Autodesk Fusion 360 part; units mm, degrees
sketch "Boceto1" plane through (0, 0, 0) normal (0, 0, 1) x (1, 0, 0)
  circle A0 centre (0, 0) radius 11.5
  line L0 (0, 0) -> (11.5, 0)
  line L1 (0, 0) -> (5.75, 9.9593)
  line L2 (0, 0) -> (-5.75, 9.9593)
  line L3 (0, 0) -> (-11.5, 0)
  line L4 (0, 0) -> (-5.75, -9.9593)
  line L5 (0, 0) -> (5.75, -9.9593)
  line L6 (5.75, 9.9593) -> (-5.75, 9.9593)
  line L7 (-5.75, 9.9593) -> (-11.5, 0)
  line L8 (-11.5, 0) -> (-5.75, -9.9593)
  line L9 (-5.75, -9.9593) -> (5.75, -9.9593)
  line L10 (5.75, -9.9593) -> (11.5, 0)
  line L11 (11.5, 0) -> (5.75, 9.9593)
  circle A1 centre (0, 0) radius 14
  dimension "d1" = 23
  dimension "d3" = 360
  dimension "d5" = 360
  dimension "d6" = 28
extrude "Extruir1" add sketch "Boceto1" along normal blind 24 contours A0 L11 | A0 L10 | A0 L6 | A0 L9 | A0 L7 | A0 L8 | A1
sketch "Boceto2" plane through (8.625, 4.9796, 0) normal (-0.866, -0.5, 0) x (0.5, -0.866, 0)
  line L0 (-5.75, 0) -> (5.75, 0)
  line L1 (5.75, 0) -> (5.75, 24)
  line L2 (5.75, 24) -> (-5.75, 24)
  line L3 (-5.75, 24) -> (-5.75, 0)
  circle A0 centre (0.25, 17) radius 4.5
  dimension "d9" = 9
  dimension "d10" = 7
  dimension "d11" = 5.5
extrude "Extruir2" cut sketch "Boceto2" along normal mid plane 54 contours A0
Design review of the part built by this model. Coordinates are the model's own, in mm. A direction names the side the tool comes from. Round coordinates to 2 decimals unless told otherwise and drop trailing zeros. Write each loop counter-clockwise with the first axis right and the second up, starting at its lowest first coordinate (ties: lowest second). Pieces come first, ordered by that corner, then holes. Notation, with made-up numbers: (37.25, 64) - (93.25, 64) arc R20 ccw to (93.25, 97) - close; hole circle Ø6 at (62, 82.25). An arc over 180 degrees is marked (long way). Return JSON: item names as keys, results as strings. Group by question number.
Item 1: The part is to be moulded in two halves that separate along X. For faces 1 (the face through (9.3, 4.2, 24)), 2 (the face through (-3.03, 13.67, 11.83)), 3 (the face through (8.665, 4.91, 9.165)), say which applies: pulls with the +X half, pulls with the -X half, needs draft (parallel to the pull), parting line crosses it, or undercut.
Item 2: We need section A-A on x = 0. Write out the cut boundary in (y, z), and give its area (3 significant figures).
Item 3: Machinability: for faces 4 (the face through (9.3, 4.2, 0)), 5 (the face through (-8.665, -4.91, 9.165)), which of the approach directions +Z, -Z, +X, -X, +Y, -Y give a long, thin tool a straight path to every point of the face, cutting with its end or side? Answer none if there is none.
Item 4: We need section C-C on y = -7. Give the number of separate pieces and of enclosed holes in the cut face, and give its area (3 significant figures).
Item 5: For probe 1 along Z at (x, y) = (9.5, 5); probe 2 along Y at (x, z) = (-6.75, 8.5); probe 3 along X at (y, z) = (-8, 22.5), list the stretches that pass through material, from the lowest coordinate up. Write a range as [from, to].
Item 6: Insertion check: P1, Ø2, axis at x = -1.5, z = 9.5, coming from the +Y side; P2, Ø5, axis at x = 9.5, z = 17, coming from the -Y side; P3, Ø12, axis at y = -5, z = 5.5, coming from the -X side; P4, Ø1, axis at x = -6, z = 17.5, coming from the -Y side. Each pin has a flat end and moves straight along its axis. Give the tip position at first contact, or say it passes through.
Item 7: We need section B-B on z = 6.25. Write out the cut boundary in (x, y).
Model answer:
{
 "1": {"face 1": "needs draft", "face 2": "parting line crosses it", "face 3": "undercut"},
 "2": {"outline": "(-14, 0) - (-9.96, 0) - (-9.96, 24) - (-14, 24) - close; (9.96, 0) - (14, 0) - (14, 24) - (9.96, 24) - close", "area": "194 mm²"},
 "3": {"face 4": "-Z, +X, -X, +Y, -Y", "face 5": "+Z, -Z"},
 "4": {"separate pieces": "3", "enclosed holes": "0", "area": "183 mm²"},
 "5": {"probe 1": "z = [0, 12.5], [21.5, 24]", "probe 2": "y = [-12.27, -8.23], [8.23, 12.27]", "probe 3": "x = [-11.49, -6.88], [6.88, 11.49]"},
 "6": {"P1": "stops at y = 13.99", "P2": "stops at y = -12.12", "P3": "stops at x = -14", "P4": "stops at y = -12.87"},
 "7": {"outline": "circle Ø28 at (0, 0); hole (-11.5, 0) - (-5.75, -9.96) - (5.75, -9.96) - (11.5, 0) - (5.75, 9.96) - (-5.75, 9.96) - close"}
}
